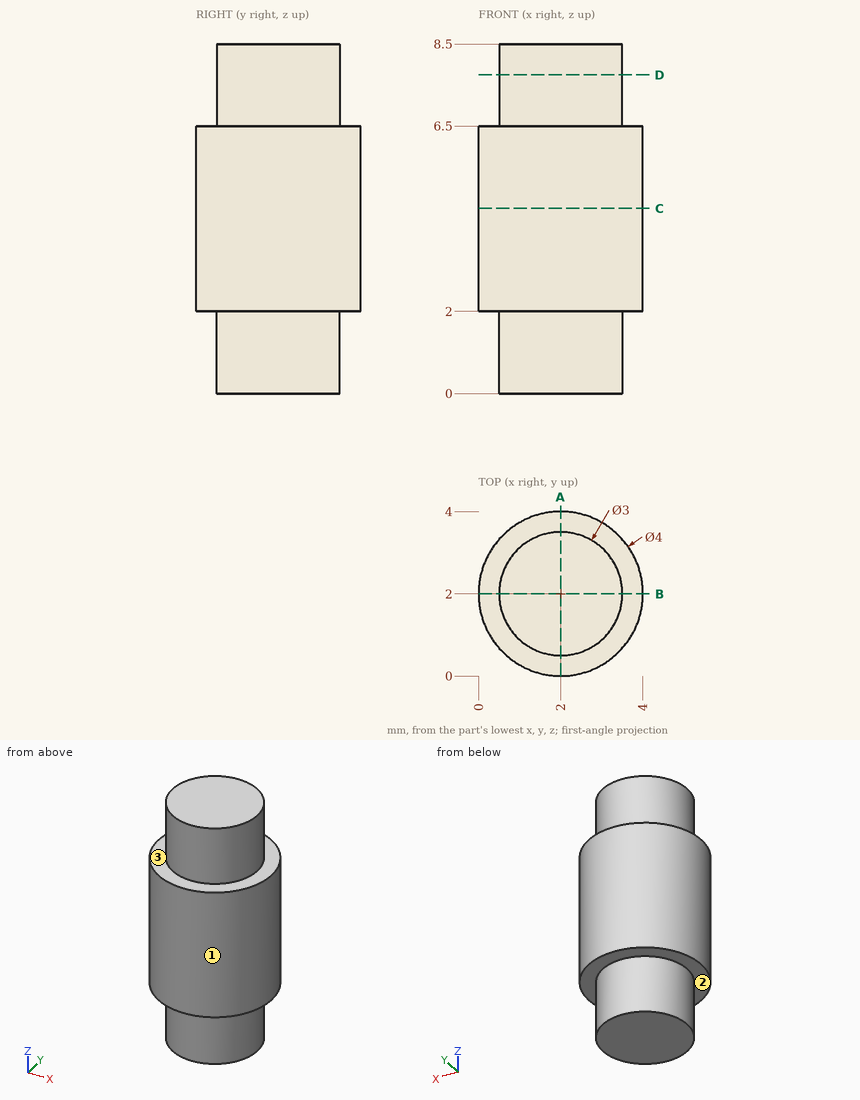
Geometry: see drawing. Coordinates: mm, zero at the bounding-box minimum. A direction names the side the tool comes from. Round coordinates to 2 decimals unless told otherwise and drop trailing zeros. Write each loop counter-clockwise with the first axis right and the second up, starting at its lowest first coordinate (ties: lowest second). Pieces come first, ordered by that corner, then holes.
1) Contact query for a flat-ended pin moving along its axis: P1, Ø1, axis at x = 2.5, z = 5.5, coming from the -Y side. Output: stop coordinate, or through.
2) Cut plane A-A (x = 2). Return the cut outline in (y, z), then the cut area to 3 significant figures.
3) Ray query, L1, parallel to Z at x = 2.65, y = 0.35; L2, parallel to Y at x = 0.3, z = 4.5; L3, parallel to X at y = 2.55, z = 1.25. Return the intervals inside material, ascending.
4) Cut plane C-C (z = 4.5). Return the cut outline in (x, y).
5) Cut plane D-D (z = 7.75). Return the cut outline in (x, y), then the cut area to 3 significant figures.
6) Reachability of the marked faces 1, 2 and 3 from +Z, -Z, +X, -X, +Y, -Y: full face, straight path, thin tool, end or side. Return the list, or none.
Geometry says:
1. P1: stops at y = 0
2. outline: (0, 2) - (0.5, 2) - (0.5, 0) - (3.5, 0) - (3.5, 2) - (4, 2) - (4, 6.5) - (3.5, 6.5) - (3.5, 8.5) - (0.5, 8.5) - (0.5, 6.5) - (0, 6.5) - close
2. area: 30.0 mm2
3. L1: z = 2 to 6.5
3. L2: y = 0.95 to 3.05
3. L3: x = 0.6 to 3.4
4. outline: circle Ø4 at (2, 2)
5. outline: circle Ø3 at (2, 2)
5. area: 7.07 mm2
6. face 1: +Z, -Z
6. face 2: -Z
6. face 3: +Z
